Can you work these out from the model? Positions are in its coordinate system, mm. A direction names the side the tool comes from. Give positions to 0.01 mm unless a question says otherwise; leave off trailing zeros. Order: outer loops, then holes, each group sorted by start corner. A loop starts at its lowest first (then second) coordinate and runs counter-clockwise, first axis right, second up. Notation, with made-up numbers: (56.5, -11.5) -> (77.5, -11.5) arc R29 cw to (77.5, 9.5) -> close; hole circle Ø3 at (69.25, 59). An arc over 180 degrees is marked (long way). Answer as a JSON object with one key per item and string values.
```python
from build123d import *

# Parameters (mm, degrees)
FILLET2_R                = 0.5
BOSS_EXTRUDE1_DEPTH      = 13.5
BOSS_EXTRUDE1_DEPTH_BACK = 13.5
SKETCH4_R                = 3.4
SKETCH2_R                = 3.7
CUT_EXTRUDE3_DEPTH       = 50
BOSS_EXTRUDE4_DEPTH      = 1
BOSS_EXTRUDE4_DEPTH_BACK = 1
FILLET10_R               = 0.3
FILLET11_R               = 0.3
FILLET12_R               = 0.3


with BuildPart() as part:
    # Sketch1 → Revolve3 (revolve)
    with BuildSketch(Plane(origin=(0, 0, 0), x_dir=(0, 0, -1), z_dir=(1, 0, 0)), mode=Mode.PRIVATE) as revolve3_sk:
        with BuildLine():
            Line((9.270955764, 5.772702061), (15.949995133, 5.772702061))
            Line((15.949995133, 5.772702061), (22.460257938, 5.405787473))
            Line((22.460257938, 5.405787473), (31.460257938, 5.405787473))
            Line((31.460257938, 5.405787473), (35.358038474, 4.669508623))
            Line((35.358038474, 4.669508623), (39.313400178, 4.15154459))
            Line((39.313400178, 4.15154459), (39.833484347, 3.774843476))
            Line((39.833484347, 3.774843476), (46.460257938, 2.972702061))
            Line((46.460257938, 2.972702061), (72.460257938, 2.972702061))
            Line((72.460257938, 2.972702061), (72.460257938, -2.027297939))
            Line((72.460257938, -2.027297939), (2.460257938, -2.027297939))
            ThreePointArc((2.460257938, -2.027297939), (4.402552529, 3.150191919), (9.270955764, 5.772702061))
        make_face()
    revolve(revolve3_sk.sketch.rotate(Axis((0, -2.027297939, -2.460257938), (0, 0, -1)), 90), axis=Axis((0, -2.027297939, -2.460257938), (0, 0, -1)))

    # Fillet2
    fillet2_edges = [part.edges().sort_by_distance(p)[0] for p in [
        (-5, -2.027297939, -46.460257938),
        (-6.696806562, -2.027297939, -35.358038474),
        (-7.433085412, -2.027297939, -31.460257938),
        (-7.433085412, -2.027297939, -22.460257938),
    ]]
    fillet(fillet2_edges, radius=FILLET2_R)

    # Sketch4 → Boss-Extrude1 (add, two sides: drawn at the far end of the back side and taken through both)
    with BuildSketch(Plane(origin=(0, 0, 0), x_dir=(0, 0, -1), z_dir=(1, 0, 0)).offset(-BOSS_EXTRUDE1_DEPTH_BACK)):
        with Locations((26.990295722, -2.027297939)):
            Circle(SKETCH4_R)
    extrude(amount=BOSS_EXTRUDE1_DEPTH + BOSS_EXTRUDE1_DEPTH_BACK)

    # Sketch2 → Cut-Extrude3 (cut)
    with BuildSketch(Plane(origin=(0, 0, -72.460257938), x_dir=(-1, 0, 0), z_dir=(0, 0, -1))):
        with Locations((0, -2.027297939)):
            Circle(SKETCH2_R)
    extrude(amount=-CUT_EXTRUDE3_DEPTH, mode=Mode.SUBTRACT)

    # Sketch5 → Boss-Extrude4 (add, two sides: drawn at the far end of the back side and taken through both)
    with BuildSketch(Plane(origin=(0, 0, 0), x_dir=(0, 0, -1), z_dir=(1, 0, 0)).offset(-BOSS_EXTRUDE4_DEPTH_BACK)):
        with BuildLine():
            Line((-0.364563148, -1.323842828), (-0.639628828, -1.177788119))
            Line((-0.639628828, -1.177788119), (-0.639628828, -2.876807758))
            Line((-0.639628828, -2.876807758), (-0.364563148, -2.730753049))
            ThreePointArc((-0.364563148, -2.730753049), (0.874853819, -3.524864677), (2.196515624, -2.876807758))
            Line((2.196515624, -2.876807758), (2.579405143, -3.3917107))
            Line((2.579405143, -3.3917107), (2.579405143, -0.662885177))
            Line((2.579405143, -0.662885177), (2.196515624, -1.177788119))
            ThreePointArc((2.196515624, -1.177788119), (0.874853819, -0.5297312), (-0.364563148, -1.323842828))
        make_face()
        with BuildLine():
            ThreePointArc((1.860257938, -2.027297939), (0.960257938, -1.127297939), (0.060257938, -2.027297939))
            ThreePointArc((0.060257938, -2.027297939), (0.960257938, -2.927297939), (1.860257938, -2.027297939))
        make_face(mode=Mode.SUBTRACT)
    extrude(amount=BOSS_EXTRUDE4_DEPTH + BOSS_EXTRUDE4_DEPTH_BACK)

    # Fillet10
    fillet10_edges = [part.edges().sort_by_distance(p)[0] for p in [
        (-1, -2.027297939, -1.860257938),
        (1, -2.027297939, -1.860257938),
    ]]
    fillet(fillet10_edges, radius=FILLET10_R)

    # Fillet11
    fillet11_edges = [part.edges().sort_by_distance(p)[0] for p in [
        (0, -2.730753049, 0.364563148),
        (0, -1.323842828, 0.364563148),
    ]]
    fillet(fillet11_edges, radius=FILLET11_R)

    # Fillet12
    fillet12_edges = [part.edges().sort_by_distance(p)[0] for p in [
        (0, -1.177788119, -2.196515624),
        (0, -2.876807758, -2.196515624),
    ]]
    fillet(fillet12_edges, radius=FILLET12_R)


solid = part.part
```
1. If we section it at D-D on z = -55: Please give me the cut outline in (x, y), then the cut area to 3 significant figures.
Worked answers:
{"outline": "circle Ø10 at (0, -2.03); hole circle Ø7.4 at (0, -2.03)", "area": "35.5 mm²"}
2. For faces 1 (the face through (3.6, 4.89, -12.66)), 2 (the face through (-0.651, -6.985, -59.657)), 3 (the face through (-0.986, -9.536, -19.974)), 4 (the face through (10.007, -1.006, -30.233)), which set-ups out of +Z, -Z, +X, -X, +Y, -Y let a thin tool reach every point of the face, with its end or its side?
Worked answers:
{"face 1": "+Z", "face 2": "-Z", "face 3": "none", "face 4": "+X"}
3. If we mould it in two halves opening along X, with no side actions, what happens to faces 5 (the face through (-0.01, -3.52, -0.81)), 6 (the face through (3.14, 4.02, -34.74)), 7 (the face through (0, -2, -22.46))? For each: +X half, -X half, draft (parallel to the pull), parting line (faces both ways), or undercut.
Worked answers:
{"face 5": "draft", "face 6": "parting line", "face 7": "undercut"}
4. If we section it at B-B on z = -5: Please give me the cut outline in (x, y).
Worked answers:
{"outline": "circle Ø11.58 at (0, -2.03)"}
5. Will these pins go through, and if not, where does the flat tip stop? pin 1 Ø3 at (y, z) = (-2.03, -0.96) entering from -X; pin 2 Ø3.5 at (x, y) = (1, -2) entering from -Z; pin 3 Ø6 at (x, z) = (-7.5, -62.5) entering from +Y.
Worked answers:
{"pin 1": "x = -1", "pin 2": "z = -22.46", "pin 3": "y = 0.15"}
6. Please list where these lines run through material, in increasing order: L1, parallel to X at y = -1.75, z = -10; L2, parallel to Z at x = 4.25, y = -2.25; L3, parallel to X at y = -3.75, z = -28.
Worked answers:
{"L1": "-7.8 to 7.8", "L2": "-72.46 to -3.71", "L3": "-13.5 to -3.27, 3.27 to 13.5"}
7. If we section it at C-C on z = -34: Please give me the cut outline in (x, y), then the cut area to 3 significant figures.
Worked answers:
{"outline": "circle Ø13.91 at (0, -2.03); hole circle Ø7.4 at (0, -2.03)", "area": "109 mm²"}
8. If we section it at A-A on z = -25.5: Please give me the cut outline in (x, y).
Worked answers:
{"outline": "(-13.5, -5.08) -> (-6.78, -5.08) arc R7.43 ccw to (6.78, -5.08) -> (13.5, -5.08) -> (13.5, 1.03) -> (6.78, 1.03) arc R7.43 ccw to (-6.78, 1.03) -> (-13.5, 1.03) -> close; hole circle Ø7.4 at (0, -2.03)"}
